Autodesk Inventor part; units mm, degrees
ref_plane "YZ Plane" through (0, 0, 0) normal (1, 0, 0) x (0, 1, 0)
ref_plane "XZ Plane" through (0, 0, 0) normal (0, 1, 0) x (-1, 0, 0)
ref_plane "XY Plane" through (0, 0, 0) normal (0, 0, 1) x (1, 0, 0)
sketch "Boceto1" plane through (0, 0, 0) normal (0, 0, 1) x (1, 0, 0)
  circle A0 centre (0, 0) radius 39
  circle A1 centre (0, 0) radius 29
  circle A2 centre (0, 0) radius 31.5
  dimension "DiametroExterior" = 78
  dimension "DiametroCaja" = 58
  dimension "d2" = 63
extrude "Extrusión1" add sketch "Boceto1" along normal blind 18 contours A2
sketch "Boceto2" plane through (0, 0, 18) normal (0, 0, 1) x (1, 0, 0)
  circle A0 centre (0, 0) radius 39
  circle A1 centre (0, 0) radius 31
  dimension "d5" = 78
  dimension "d6" = 62
extrude "Extrusión2" add sketch "Boceto2" against normal blind 3
sketch "Boceto3" plane through (0, 0, 0) normal (0, 0, -1) x (-1, 0, 0)
  circle A0 centre (0, 0) radius 29
  dimension "d9" = 58
extrude "Extrusión3" add sketch "Boceto3" against normal blind 6
sketch "Boceto5" plane through (0, 0, 15) normal (0, 0, -1) x (-1, 0, 0)
  line L0 (0, 0) -> (33, 0) construction
  line L1 (0, 0) -> (33.75, 0) construction
  circle A0 centre (0, 0) radius 39
  circle A1 centre (0, 0) radius 31.5
  circle A2 centre (25.1022, 25.1024) radius 2
  circle A3 centre (25.1024, -25.1022) radius 2
  circle A4 centre (-25.1022, -25.1024) radius 2
  circle A5 centre (-25.1024, 25.1022) radius 2
  point P0 (23.8649, 23.8649)
  dimension "d14" = 33.75
  dimension "d81" = 78
  dimension "d82" = 63
  dimension "d83" = 4
  dimension "d84" = 2
  dimension "d85" = 1.5
  dimension "d86" = 360
sketch "Boceto6" plane through (0, 0, 6) normal (0, 0, 1) x (1, 0, 0)
  line L0 (-16, -25) -> (16, -25)
  line L1 (16, -25) -> (16, 25)
  line L2 (16, 25) -> (-16, 25)
  line L3 (-16, 25) -> (-16, -25)
  line L4 (-16, -25) -> (16, 25) construction
  line L5 (16, -25) -> (-16, 25) construction
  circle A0 centre (0, 13.5) radius 12.5
  circle A1 centre (-8, -22.5) radius 1.1
  circle A2 centre (8, -22.5) radius 1.1
  circle A3 centre (13.5, -17) radius 1.1
  circle A4 centre (-13.5, -17) radius 1.1
  circle A5 centre (-13.5, -9) radius 1.1
  circle A6 centre (-13.5, -1) radius 1.1
  circle A7 centre (-13.5, 7) radius 1.1
  circle A8 centre (13.5, 7) radius 1.1
  circle A9 centre (13.5, -1) radius 1.1
  circle A10 centre (13.5, -9) radius 1.1
  line L6 (0, -25) -> (0, -19)
  line L7 (0, -19) -> (-8.307, -19)
  line L8 (0, -19) -> (8.307, -19)
  line L9 (-11.657, -15.65) -> (-11.657, 6.356)
  line L10 (11.657, -15.65) -> (11.657, 6.356)
  line L11 (10.857, 7.156) -> (9.815, 7.156)
  line L12 (-10.857, 7.156) -> (-9.815, 7.156)
  arc A11 (-9.015, 6.356) -> (9.015, 6.356) centre (0, 13.002) ccw
  arc A12 (9.815, 7.156) -> (9.015, 6.356) centre (9.815, 6.356) ccw
  arc A13 (11.657, 6.356) -> (10.857, 7.156) centre (10.857, 6.356) ccw
  arc A14 (-9.015, 6.356) -> (-9.815, 7.156) centre (-9.815, 6.356) ccw
  arc A15 (-10.857, 7.156) -> (-11.657, 6.356) centre (-10.857, 6.356) ccw
  arc A16 (10.857, -16.45) -> (11.657, -15.65) centre (10.857, -15.65) ccw
  arc A17 (10.857, -16.45) -> (9.107, -18.2) centre (10.857, -18.2) ccw
  arc A18 (8.307, -19) -> (9.107, -18.2) centre (8.307, -18.2) ccw
  arc A19 (-9.107, -18.2) -> (-8.307, -19) centre (-8.307, -18.2) ccw
  arc A20 (-9.107, -18.2) -> (-10.857, -16.45) centre (-10.857, -18.2) ccw
  arc A21 (-11.657, -15.65) -> (-10.857, -16.45) centre (-10.857, -15.65) ccw
  point P0 (0, 0)
  point P1 (0, 0)
  point P2 (10.7705, 7.156)
  point P3 (-10.7705, 7.156)
  point P4 (4.899, 25)
  point P5 (-4.899, 25)
  dimension "d27" = 32
  dimension "d28" = 50
  dimension "d29" = 25
  dimension "d30" = 11.5
  dimension "d31" = 2.2
  dimension "d32" = 2.2
  dimension "d33" = 2.2
  dimension "d34" = 2.2
  dimension "d35" = 2.2
  dimension "d36" = 2.2
  dimension "d37" = 2.2
  dimension "d38" = 2.2
  dimension "d39" = 2.2
  dimension "d40" = 2.2
  dimension "d41" = 27
  dimension "d42" = 16
  dimension "d43" = 36
  dimension "d44" = 30.5
  dimension "d45" = 6.5
  dimension "d46" = 8
  dimension "d47" = 8
  dimension "d48" = 8
  dimension "d49" = 8
  dimension "d50" = 8
  dimension "d51" = 8
  dimension "d52" = 6
  dimension "d53" = 8.307
  dimension "d54" = 22.006
  dimension "d55" = 1.042
  dimension "d56" = 1.042
  dimension "d57" = 11.2
  dimension "d58" = 0.8
  dimension "d59" = 0.8
  dimension "d60" = 0.8
  dimension "d61" = 0.8
  dimension "d62" = 1.75
  dimension "d63" = 0.8
  dimension "d64" = 1.75
  dimension "d65" = 0.8
extrude "Extrusión4" cut sketch "Boceto6" against normal blind 3 contours L7 A19 A20 A21 L9 A15 L12 A0 L11 A13 L10 A16 A17 A18 L8
hole "Agujero2" at (13.5, -17, 6) at (13.5, -9, 6) at (8, -22.5, 6) at (-8, -22.5, 6) at (-13.5, -9, 6) at (-13.5, -17, 6) direction (0, 0, -1) diameter 2.013 depth 7.6
extrude "Extrusión6" cut sketch "Boceto6" against normal blind 6 contours A0 L2 | L2 A0 L11 A12 A11 A14 L12 | L12 A14 A11 A12 L11 A0
hole "Agujero3" at (-25.1022, 25.1024, 15) at (25.1024, 25.1022, 15) at (25.1022, -25.1024, 15) at (-25.1024, -25.1022, 15) direction (0, 0, 1) diameter 2.85 depth 10.4 counterbore diameter 6 counterbore depth 2
sketch "Boceto7" plane through (0, 0, 0) normal (0, 0, -1) x (-1, 0, 0)
  arc A0 (-10.7705, 7.156) -> (10.7705, 7.156) centre (0, 13.5) ccw
  line L0 (0, 26) -> (0, 13.5)
  circle A1 centre (0, 13.5) radius 20.6175
  circle A2 centre (0, 13.5) radius 24.6175
  point P0 (0, 0)
  dimension "DiametroRodamiento" = 41.235
  dimension "d97" = 49.235
extrude "Extrusión7" add sketch "Boceto7" along normal blind 28.934
sketch "Boceto8" plane through (0, 0, 0) normal (0, 0, -1) x (-1, 0, 0)
  circle A0 centre (0, 0) radius 31.5
  circle A1 centre (0, 0) radius 31.5
  circle A2 centre (0, 13.5) radius 24.6175
  circle A3 centre (0, 13.5) radius 20.6175
  point P0 (23.4296, 21.0548)
  point P1 (-23.4296, 21.0548)
extrude "Extrusión8" add sketch "Boceto8" against normal blind 15 contours A0 A3 A2 | A0 A3 picked at (0.7908, 36.6312) picked at (3.3504, 32.0101)
sketch "Boceto9" plane through (0, 13.5, 0) normal (0, 0, -1) x (-1, 0, 0)
  circle A0 centre (0, 0) radius 12.5
  circle A1 centre (0, 0) radius 20.6175
  point P0 (0, -13.5)
extrude "Extrusión9" add sketch "Boceto9" along normal blind 6
equation "\"d5\" = DiametroExterior"
equation "\"d9\" = DiametroCaja"
equation "\"d83\" = d87"
equation "\"d31\" = d37"
equation "\"d32\" = d37"
equation "\"d33\" = d37"
equation "\"d35\" = d37"
equation "\"d36\" = d37"
equation "\"d38\" = d37"
equation "\"d39\" = d37"
equation "\"d40\" = d37"
equation "\"d47\" = d46"
equation "\"d48\" = d46"
equation "\"d49\" = d46"
equation "\"d50\" = d46"
equation "\"d51\" = d46"
properties part number "B-03" material "PETG"
Design review of the part built by this model. Coordinates are the model's own, in mm. A direction names the side the tool comes from. Coordinates: 2 decimals unless noted, no trailing zeros. Order: outer loops, then holes, each group sorted by start corner. A loop starts at its lowest first (then second) coordinate and runs counter-clockwise, first axis right, second up. Notation, with made-up numbers: (1, -9) -> (39, -9) arc R26 ccw to (39, 23) -> close; hole circle Ø1 at (-33.75, -22). An arc over 180 degrees is marked (long way). One line per item, written item: value. Start each with the question number.
Q1. Mouldability with a two-part tool opening along X and no side actions: class faces 4 (the flat face through (-29, -3, 18)), 5 (the flat face through (-12, 0, 6)), 6 (the cylindrical face through (-5.077, 38.668, 16.521)) as pulls with the +X half, pulls with the -X half, needs draft (parallel to the pull), parting line crosses it, or undercut.
Q2. Take a section at D-D, the plane z = -11. State the section outline as (x, y) points (1 decimal).
Q3. For probe 1 along X at (y, z) = (-9, 1.35); probe 2 along Y at (x, z) = (8, 3.3); probe 3 along Z at (x, y) = (-16, 22), list the stretches that pass through material, from the lowest coordinate up.
Q4. Tool access review of faces 1 (the flat face through (0, -19, 5)), 2 (the flat face through (0, -32, 15)), 3 (the cylindrical face through (7.956, -21.494, 2.958)): name each direction out of +Z, -Z, +X, -X, +Y, -Y from which nothing blocks a thin tool from reaching the whole face with its end or side.
Q5. Take a section at A-A, the plane x = 0. State the section outline as (y, z) points.
Q6. Take a section at C-C, the plane x = 13.5. State the section outline as (y, z) points, then the cut area to 3 significant figures.
Q7. Take a section at B-B, the plane y = 12. State the section outline as (x, z) points.
Q8. Insertion check: pin 1 Ø1 at (x, z) = (-17.5, -3) entering from -Y; pin 2 Ø3.5 at (y, z) = (-9, 4.5) entering from +X; pin 3 Ø5 at (x, y) = (24, 26.5) entering from -Z; pin 4 Ø8 at (x, y) = (-25.1, -25.1) entering from +Z. Each pin has a flat end and moves straight along its axis. Give the tip position at first contact, or say it passes through.
Values follow:
1. face 4: needs draft
1. face 5: undercut
1. face 6: parting line crosses it
2. outline: circle Ø49.2 at (0, 13.5); hole circle Ø41.2 at (0, 13.5)
3. probe 1: x = -30.19 to -14.51, -12.49 to 12.49, 14.51 to 30.19
3. probe 2: y = -30.47 to -23.51, -21.49 to -19, 23.1 to 36.78
3. probe 3: z = -6 to 6
4. face 1: +Z
4. face 2: -Z
4. face 3: +Z, -Z
5. outline: (-39, 15) -> (-31.5, 15) -> (-31.5, 0) -> (-11.12, 0) -> (-11.12, -28.93) -> (-7.12, -28.93) -> (-7.12, -6) -> (1, -6) -> (1, 3) -> (-19, 3) -> (-19, 6) -> (-29, 6) -> (-29, 18) -> (-39, 18) -> close; (26, -6) -> (34.12, -6) -> (34.12, -28.93) -> (38.12, -28.93) -> (38.12, 15) -> (39, 15) -> (39, 18) -> (29, 18) -> (29, 6) -> (26, 6) -> close
6. outline: (-36.59, 15) -> (-28.46, 15) -> (-28.46, 0) -> (-18.01, 0) -> (-18.01, 6) -> (-25.67, 6) -> (-25.67, 18) -> (-36.59, 18) -> close; (-15.99, 0) -> (-10.01, 0) -> (-10.01, 6) -> (-15.99, 6) -> close; (-7.99, 0) -> (-7.09, 0) -> (-7.09, -28.93) -> (-2.08, -28.93) -> (-2.08, -6) -> (29.08, -6) -> (29.08, -28.93) -> (34.09, -28.93) -> (34.09, 15) -> (36.59, 15) -> (36.59, 18) -> (25.67, 18) -> (25.67, 6) -> (-7.99, 6) -> close
6. area: 994 mm2
7. outline: (-37.11, 15) -> (-29.12, 15) -> (-29.12, 0) -> (-24.57, 0) -> (-24.57, -28.93) -> (-20.56, -28.93) -> (-20.56, -6) -> (-12.41, -6) -> (-12.41, 6) -> (-26.4, 6) -> (-26.4, 18) -> (-37.11, 18) -> close; (12.41, -6) -> (20.56, -6) -> (20.56, -28.93) -> (24.57, -28.93) -> (24.57, 0) -> (29.12, 0) -> (29.12, 15) -> (37.11, 15) -> (37.11, 18) -> (26.4, 18) -> (26.4, 6) -> (12.41, 6) -> close
8. pin 1: stops at y = -4.31
8. pin 2: stops at x = 30.65
8. pin 3: stops at z = 15
8. pin 4: stops at z = 18
